The listing builds one solid part. Answer for the finished solid, in the listing's coordinates (mm). A direction names the side the tool comes from. Round coordinates to 2 decimals unless told otherwise and drop trailing zeros. Loops run counter-clockwise (first coordinate to the right, second up) from the corner with the lowest first, then second, coordinate; pieces in that order, holes last. Notation, with made-up numbers: (45.5, 55) -> (55.5, 55) arc R20 ccw to (55.5, 61) -> close; hole circle Ø5 at (27.5, -13). An arc over 180 degrees is marked (long way). One line per question, with ' | ' between items.
from build123d import *

# Parameters (mm, degrees)
F1_DEPTH = 150
F2_R     = 40
F3_DEPTH = 40
F4_R     = 20
F5_DEPTH = 70.001


with BuildPart() as f1:
    # F0 (on Front) → F1 (new body)
    with BuildSketch(Plane.XZ):
        Polygon((0, 70), (0, 0), (125, 0), (125, 30), (53.094011, 30), (30, 70), align=None)
    extrude(amount=-F1_DEPTH)

    # F2 (on face) → F3 (join, through all)
    with BuildSketch(Plane.XY.offset(70)):
        with Locations((50, 75)):
            Circle(F2_R)
    extrude(amount=-F3_DEPTH)

    # F4 (on face) → F5 (cut, through all)
    with BuildSketch(Plane.XY.offset(70)):
        with Locations((50, 75)):
            Circle(F4_R)
    extrude(amount=-F5_DEPTH, mode=Mode.SUBTRACT)


solid = f1.part
Q1. For faces 4 (the face through (98, 74, 30)), 5 (the face through (48, 150, 28)), determine the directions among +Z, -Z, +X, -X, +Y, -Y from which every point of the face is accessible in a straight line to the end or side of a thin tool.
Numbers:
face 4: +Z, +X | face 5: +Z, -Z, +X, -X, +Y
Q2. Find the intervals of material crossed by line 1 (Y direction, x = 50, z = 22); line 2 (Y direction, x = 50, z = 37); line 3 (Z direction, x = 99.5, y = 54.5), in increasing order. Write a range as from..to.
Numbers:
line 1: 0..55, 95..150 | line 2: 35..55, 95..115 | line 3: 0..30
Q3. A cutting plane is placed at B-B on y = 75. Give the vertices of the cut face in (x, z).
Numbers:
outline: (0, 0) -> (30, 0) -> (30, 70) -> (0, 70) -> close; (70, 0) -> (125, 0) -> (125, 30) -> (90, 30) -> (90, 70) -> (70, 70) -> close
Q4. Given pin 1 Ø5 at (y, z) = (66, 59.5) entering from +X, flat-ended and moving along its own axis, determine where the tip first touches the part or whether it passes through.
Numbers:
pin 1: x = 89.47
Q5. A cutting plane is placed at C-C on z = 37. Give the vertices of the cut face in (x, y).
Numbers:
outline: (0, 0) -> (49.05, 0) -> (49.05, 35.01) arc R40 ccw (long way) to (49.05, 114.99) -> (49.05, 150) -> (0, 150) -> close; hole circle Ø40 at (50, 75)
Q6. A cutting plane is placed at D-D on y = 131.5. Give the vertices of the cut face in (x, z), plus the area to 3 significant figures.
Numbers:
outline: (0, 0) -> (125, 0) -> (125, 30) -> (53.09, 30) -> (30, 70) -> (0, 70) -> close | area: 5,410 mm^2
Q7. A cutting plane is placed at A-A on x = 32. Give the vertices of the cut face in (y, z), plus the area to 3 significant figures.
Numbers:
outline: (0, 0) -> (66.28, 0) -> (66.28, 70) -> (39.28, 70) -> (39.28, 66.54) -> (0, 66.54) -> close; (83.72, 0) -> (150, 0) -> (150, 66.54) -> (110.72, 66.54) -> (110.72, 70) -> (83.72, 70) -> close | area: 9,010 mm^2
Q8. For a pull along Y with two mould halves and no side action, classify faces 1 (the face through (59.229, 57.257, 35.49)), 2 (the face through (41.71, 19.9, 49.72)), 3 (the face through (48, 0, 28)) as pulls with the +Y half, pulls with the -Y half, needs draft (parallel to the pull), parting line crosses it, or undercut.
Numbers:
face 1: undercut | face 2: needs draft | face 3: pulls with the -Y half
